The model under review builds one solid part; all positions refer to its coordinate system, in mm. A direction names the side the tool comes from. Round coordinates to 2 decimals unless told otherwise and drop trailing zeros. Order: outer loops, then holes, each group sorted by start corner. A loop starts at its lowest first (then second) coordinate and runs counter-clockwise, first axis right, second up.
Autodesk Inventor part; units mm, degrees
ref_plane "YZ Plane" through (0, 0, 0) normal (1, 0, 0) x (0, 1, 0)
ref_plane "XZ Plane" through (0, 0, 0) normal (0, 1, 0) x (-1, 0, 0)
ref_plane "XY Plane" through (0, 0, 0) normal (0, 0, 1) x (1, 0, 0)
sketch "Sketch1" plane through (0, 0, 0) normal (0, 0, 1) x (1, 0, 0)
  arc A0 (-1.1319, 20.1168) -> (-1.6326, 25.8318) centre (16.7386, 24.5618) ccw
  line L0 (0, 0) -> (33.4772, 0)
  line L1 (33.4772, 0) -> (33.4772, 11.955)
  line L2 (0, 0) -> (0, 11.955)
  line L3 (-1.2219, 13.7668) -> (-11.2014, 13.7668)
  line L4 (-11.2014, 13.7668) -> (-11.2014, 20.1168)
  line L5 (-11.2014, 20.1168) -> (-1.1319, 20.1168)
  line L6 (-11.2014, 25.8318) -> (-1.6326, 25.8318)
  line L7 (-11.2014, 25.8318) -> (-11.2014, 29.0068)
  line L8 (-11.2014, 29.0068) -> (3.6223, 40.9042)
  arc A1 (-1.2219, 13.7668) -> (0, 11.955) centre (16.7386, 24.5618) ccw
  arc A2 (33.4772, 11.955) -> (3.6223, 40.9042) centre (16.7386, 24.5618) ccw
  dimension "d0" = 24.5618
  dimension "d1" = 16.7386
  dimension "d2" = 36.83
  dimension "d4" = 33.4772
  dimension "d5" = 11.955
  dimension "d6" = 6.35
  dimension "d7" = 13.7668
  dimension "d8" = 5.715
  dimension "d9" = 27.94
  dimension "d10" = 3.175
  dimension "d13" = 20.955
extrude "Clamp Body" add sketch "Sketch1" along normal blind 11.43
sketch "Sketch2" plane through (0, 0, 0) normal (0, -1, 0) x (1, 0, 0)
  circle A0 centre (3.2512, 5.715) radius 1.5
  circle A1 centre (30.2006, 5.715) radius 1.5
  line L0 (-11.2014, 0) -> (-1.2219, 0)
  line L1 (0, 0) -> (0, 11.43)
  line L2 (33.4772, 0) -> (33.4772, 11.43)
  dimension "d16" = 3
  dimension "d17" = 5.715
  dimension "d18" = 26.9494
  dimension "d20" = 3.2512
  dimension "d21" = 3.2766
hole "Mounting Holes" at (30.2006, 0, 5.715) at (3.2512, 0, 5.715) direction (0, 1, 0) diameter 3 depth 9.525 tip angle 118 countersink diameter 4 countersink angle 90
sketch "Sketch7" plane through (-11.2014, 20.1168, 0) normal (0, 1, 0) x (1, 0, 0)
  circle A0 centre (5.08, -5.715) radius 1.5
  line L0 (0, 0) -> (0, -11.43)
  line L1 (10.0695, 0) -> (0, 0)
  point P0 (11.2014, 0)
  dimension "d41" = 3
  dimension "d42" = 5.08
  dimension "d43" = 5.715
hole "Tightner Threaded Hole" at (-6.1214, 20.1168, 5.715) direction (0, -1, 0) diameter 3 end through all countersink diameter 4 countersink angle 90
sketch "Sketch4" plane through (-11.2014, 25.8318, 0) normal (0, -1, 0) x (1, 0, 0)
  circle A0 centre (5.08, 5.715) radius 1.95
  circle A1 centre (5.08, 5.715) radius 1.5
  point P0 (11.2014, 0)
  dimension "d31" = 3.9
extrude "Tightner Hole" cut sketch "Sketch4" against normal blind 9.525 contours A0 | A1
sketch "Sketch6" plane through (-11.2014, 25.8318, 0) normal (-1, 0, 0) x (0, 0, 1)
  line L0 (2.413, 3.175) -> (9.017, 3.175)
  line L1 (9.017, 3.175) -> (9.017, 15.875)
  line L2 (9.017, 15.875) -> (2.413, 15.875)
  line L3 (2.413, 15.875) -> (2.413, 3.175)
  line L4 (0, 3.175) -> (0, 0)
  line L5 (11.43, 3.175) -> (11.43, 0)
  line L6 (0, 3.175) -> (11.43, 3.175)
  point P0 (0, -25.8318)
  dimension "d34" = 2.413
  dimension "d35" = 2.413
  dimension "d36" = 12.7
  dimension "d39" = 6.604
extrude "Tightner Cutout" cut sketch "Sketch6" against normal blind 8.89
fillet "Tightner Fillet" radius 3.175 2 edges at (-2.3114, 32.5743, 2.413) (-2.3114, 32.5743, 9.017)
properties part number "MotorClampXT"
(1) Insertion check: pin 1 (5 mm diameter, centred on x = 24.5, z = 7, fed in from +Y); pin 2 (2.5 mm diameter, centred on x = -6.12, z = 5.72, fed in from -Y); pin 3 (1.5 mm diameter, centred on x = 9.5, z = 1, fed in from -Y); pin 4 (3 mm diameter, centred on y = 39.5, z = 10, fed in from +X). Each pin has a flat end and moves straight along its axis. Give the tip position at first contact, or say it passes through.
Data:
pin 1: stops at y = 44.85
pin 2: passes through
pin 3: stops at y = 0
pin 4: stops at x = 32.82
(2) Consider section A-A (x = -3.5). Write out the cut boundary in (y, z), and give its area (3 significant figures).
Data:
outline: (13.77, 0) - (20.12, 0) - (20.12, 11.43) - (13.77, 11.43) - close; (25.83, 0) - (35.19, 0) - (35.19, 3.11) - (29.01, 3.11) - (29.01, 8.32) - (35.19, 8.32) - (35.19, 11.43) - (25.83, 11.43) - close
area: 147 mm2
(3) Consider section C-C (z = 9.75). Write out the cut boundary in (x, y) (3 decimals), and give its area (3 significant figures).
Data:
outline: (-11.201, 13.767) - (-1.222, 13.767) arc R20.96 ccw to (0, 11.955) - (0, 0) - (33.477, 0) - (33.477, 11.955) arc R20.955 ccw to (3.622, 40.904) - (-11.201, 29.007) - (-11.201, 25.832) - (-1.633, 25.832) arc R18.415 cw (long way) to (-1.132, 20.117) - (-11.201, 20.117) - close
area: 615 mm2
(4) Consider section D-D (y = 5.5). Write out the cut boundary in (x, z) (3 decimals).
Data:
outline: (0, 0) - (33.477, 0) - (33.477, 11.43) - (0, 11.43) - close; hole circle Ø3 at (3.251, 5.715); hole circle Ø3 at (30.201, 5.715)
(5) Consider section B-B (y = 39). Write out the cut boundary in (x, z), and give its area (3 significant figures).
Data:
outline: (1.25, 0) - (5.31, 0) - (5.31, 11.43) - (1.25, 11.43) - close; (28.17, 0) - (31.93, 0) - (31.93, 11.43) - (28.17, 11.43) - close
area: 89.3 mm2
(6) For faces 1 (the cylindrical face through (2.801, 5.076, 4.284)), 2 (the cylindrical face through (-3.266, 32.524, 3.318)), 3 (the flat face through (-7, 13.767, 4)), 4 (the cylindrical face through (-7.67, 27.4, 4.53)), 5 (the flat face through (-8, 25.832, 4)), list the 3-axis set-ups (+Z, -Z, +X, -X, +Y, -Y) from which the entire face can be reached by the end or side of a thin tool; tool diameter is ignored.
Data:
face 1: -Y
face 2: -X, +Y
face 3: +Z, -Z, -X, -Y
face 4: +Y
face 5: +Z, -Z, -X
(7) Draft analysis for pull direction Z (two halves, no side actions). For faces 6 (the flat face through (6, 9, 11.43)), 7 (the flat face through (-7, 30, 9.017)), 8 (the flat face through (-11.201, 27, 6)), state which applies: pulls with the +Z half, pulls with the -Z half, needs draft (parallel to the pull), parting line crosses it, or undercut.
Data:
face 6: pulls with the +Z half
face 7: undercut
face 8: needs draft
(8) To check wall thickness, follow probe 1 along Y at (x, z) = (16.5, 3.25); probe 2 along Y at (x, z) = (-5, 3.5); probe 3 along X at (y, z) = (38.5, 3). State the ranges of each line that lie inside material, in increasing order.
Data:
probe 1: y = 0 to 6.15, 42.98 to 45.52
probe 2: y = 13.77 to 20.12, 25.83 to 29.01
probe 3: x = 0.63 to 4.7, 28.77 to 32.39
